from build123d import *

# Parameters (mm, degrees)
SKETCH2_R           = 5.05
SKETCH2_R_2         = 4.05
SKETCH2_R_3         = 2
BOSS_EXTRUDE1_DEPTH = 10


with BuildPart() as part:
    # Sketch2 → Boss-Extrude1 (new body)
    with BuildSketch(Plane.XY):
        with BuildLine():
            Line((-52.525602652, 39.073613719), (55.40832582, 23.904489319))
            Line((55.40832582, 23.904489319), (88.545070057, 37.292603029))
            ThreePointArc((88.545070057, 37.292603029), (113.24947567, 26.806204997), (102.763077638, 2.101799383))
            Line((102.763077638, 2.101799383), (56.40388491, -16.628530288))
            Line((56.40388491, -16.628530288), (-52.525602652, -1.319489182))
            Line((-52.525602652, -1.319489182), (-84.855091861, -14.38145069))
            ThreePointArc((-84.855091861, -14.38145069), (-109.23231099, -4.033935081), (-98.88479538, 20.343284048))
            Line((-98.88479538, 20.343284048), (-52.525602652, 39.073613719))
        make_face()
        with Locations((-91.869943621, 2.980916679)):
            Circle(SKETCH2_R, mode=Mode.SUBTRACT)
        with Locations((95.654073847, 19.697201206)):
            Circle(SKETCH2_R_2, mode=Mode.SUBTRACT)
        with Locations((-52.525602652, 33.073613719)):
            Circle(SKETCH2_R_3, mode=Mode.SUBTRACT)
        with Locations((55.555695905, 17.904489319)):
            Circle(SKETCH2_R_3, mode=Mode.SUBTRACT)
        with Locations((-52.525602652, 4.680510818)):
            Circle(SKETCH2_R_3, mode=Mode.SUBTRACT)
        with Locations((56.256514825, -10.628530288)):
            Circle(SKETCH2_R_3, mode=Mode.SUBTRACT)
        with BuildLine():
            Line((-33.124360513, 22.209360939), (-11.338463, 19.147552718))
            ThreePointArc((-11.338463, 19.147552718), (-6.231893194, 12.3709057), (-13.008540212, 7.264335893))
            Line((-13.008540212, 7.264335893), (-34.794437724, 10.326144114))
            ThreePointArc((-34.794437724, 10.326144114), (-39.901007531, 17.102791132), (-33.124360513, 22.209360939))
        make_face(mode=Mode.SUBTRACT)
        with BuildLine():
            Line((-78.505415838, 13.773210112), (-67.379209583, 18.268489233))
            ThreePointArc((-67.379209583, 18.268489233), (-60.870257343, 15.505602928), (-63.633143649, 8.996650688))
            Line((-63.633143649, 8.996650688), (-74.759349904, 4.501371567))
            ThreePointArc((-74.759349904, 4.501371567), (-81.268302144, 7.264257873), (-78.505415838, 13.773210112))
        make_face(mode=Mode.SUBTRACT)
        with BuildLine():
            Line((67.013646361, 13.518391096), (78.139852616, 18.013670217))
            ThreePointArc((78.139852616, 18.013670217), (84.648804856, 15.250783911), (81.88591855, 8.741831672))
            Line((81.88591855, 8.741831672), (70.759712296, 4.246552551))
            ThreePointArc((70.759712296, 4.246552551), (64.250760056, 7.009438856), (67.013646361, 13.518391096))
        make_face(mode=Mode.SUBTRACT)
        with BuildLine():
            Line((16.389042924, 15.250705891), (38.174940437, 12.18889767))
            ThreePointArc((38.174940437, 12.18889767), (43.281510244, 5.412250652), (36.504863225, 0.305680845))
            Line((36.504863225, 0.305680845), (14.718965713, 3.367489066))
            ThreePointArc((14.718965713, 3.367489066), (9.612395906, 10.144136084), (16.389042924, 15.250705891))
        make_face(mode=Mode.SUBTRACT)
    extrude(amount=BOSS_EXTRUDE1_DEPTH)


solid = part.part
The listing builds one solid part. Answer for the finished solid, in the listing's coordinates (mm). A direction names the side the tool comes from. Coordinates: 2 decimals unless noted, no trailing zeros. Loops run counter-clockwise (first coordinate to the right, second up) from the corner with the lowest first, then second, coordinate; pieces in that order, holes last.
1) Find section A-A on x = -25. Write down the section's boundary in (y, z).
2) Find the intervals of material crossed by L1, parallel to Y at x = -51, z = 2.75; L2, parallel to X at y = 5, z = 8.5; L3, parallel to Y at x = 23.5, z = 2.75, in increasing order.
3) Determine the mould class of faces 3 (the face through (4, 12, 0)), 4 (the face through (-68.464, -7.759, 4.93)), 5 (the face through (72.499, 15.735, 4.93)) for opening direction Y: pulls with the +Y half, pulls with the -Y half, needs draft (parallel to the pull), parting line crosses it, or undercut.
4) A tool of negligible diameter and unlimited length cuts with its end or side. For faces 1 (the face through (43.3, 5.54, 4.93)), 2 (the face through (79.91, -7.13, 4.93)), from which of +Z, -Z, +X, -X, +Y, -Y can it reach the whole face along a straight path? Write none if from no direction.
5) Flat-ended cylindrical pins translate along their axes: pin 1 Ø2 at (x, z) = (-45.5, 1.5) entering from -Y; pin 2 Ø2 at (y, z) = (17.5, 4) entering from +X; pin 3 Ø3 at (x, z) = (-48.5, 8) entering from +Y. Find the tip coordinate at first contact, or state that the pin passes through.
6) Find section C-C on y = 29. Write down the section's boundary in (x, z), then the cut area to 3 significant figures.
7) Find section B-B on z = 2.25. Give the number of separate pieces and of enclosed holes in the cut face, then the cut area to 3 significant figures.
Values:
1. outline: (-5.19, 0) - (8.95, 0) - (8.95, 10) - (-5.19, 10) - close; (21.07, 0) - (35.21, 0) - (35.21, 10) - (21.07, 10) - close
2. L1: y = -1.53 to 3.39, 5.97 to 31.78, 34.37 to 38.86
2. L2: x = -110.49 to -96.5, -87.24 to -79.44, -73.53 to -54.5, -50.55 to 11.38, 43.21 to 65.74, 72.62 to 107.66
2. L3: y = -12 to 2.13, 14.25 to 28.39
3. face 3: needs draft
3. face 4: pulls with the -Y half
3. face 5: undercut
4. face 1: +Z, -Z
4. face 2: +Z, -Z, +X, -Y
5. pin 1: stops at y = -2.45
5. pin 2: stops at x = 114.59
5. pin 3: stops at y = 38.72
6. outline: (-77.46, 0) - (19.15, 0) - (19.15, 10) - (-77.46, 10) - close; (68.02, 0) - (112.19, 0) - (112.19, 10) - (68.02, 10) - close
6. area: 1,410 mm2
7. separate pieces: 1
7. enclosed holes: 10
7. area: 7,380 mm2
